```python
from build123d import *

# Parameters (mm, degrees)
F3_DEPTH = 82.392052


with BuildPart() as f1:
    # F0 (on Front) → F1 (revolve)
    with BuildSketch(Plane.XZ):
        with BuildLine():
            Line((-57.507594, 8), (-62.5, 8))
            Line((-62.5, 8), (-62.5, 0))
            Line((-62.5, 0), (-20.108948, 0))
            Line((-20.108948, 0), (19.891052, 0))
            Line((19.891052, 0), (62.5, 0))
            Line((62.5, 0), (62.5, 8))
            Line((62.5, 8), (57.492453, 8))
            Line((57.492453, 8), (57.492453, 5))
            Line((57.492453, 5), (52.492453, 5))
            Line((52.492453, 5), (52.492453, 8))
            Line((52.492453, 8), (19.891052, 8))
            Line((19.891052, 8), (19.891052, 96))
            ThreePointArc((19.891052, 96), (18.426586, 99.535534), (14.891052, 101))
            Line((14.891052, 101), (-15.108948, 101))
            ThreePointArc((-15.108948, 101), (-18.644481, 99.535534), (-20.108948, 96))
            Line((-20.108948, 96), (-20.108948, 8))
            Line((-20.108948, 8), (-52.507594, 8))
            Line((-52.507594, 8), (-52.507594, 5))
            Line((-52.507594, 5), (-57.507594, 5))
            Line((-57.507594, 5), (-57.507594, 8))
        make_face()
    revolve(axis=Axis((-6.764503, 0, 0), (1, 0, 0)))

    # F2 (on face) → F3 (cut, through all)
    with BuildSketch(Plane.YZ.offset(19.891052)):
        with BuildLine():
            Line((-9.635893, 76.123558), (-1.004641, 7.936668))
            ThreePointArc((-1.004641, 7.936668), (0, 8), (1.004641, 7.936668))
            Line((1.004641, 7.936668), (9.635893, 76.123558))
            Line((9.635893, 76.123558), (0, 76.123558))
            Line((0, 76.123558), (-9.635893, 76.123558))
        make_face()
    extrude(amount=-F3_DEPTH, mode=Mode.SUBTRACT)


solid = f1.part
```
CAD build for the part. Positions are in the model's coordinates, mm. A direction names the side the tool comes from. Coordinates: 2 decimals unless noted, no trailing zeros. Loops run counter-clockwise (first coordinate to the right, second up) from the corner with the lowest first, then second, coordinate; pieces in that order, holes last. Notation, with made-up numbers: (-40, -35) - (-33, -35) arc R27 cw to (-33, -10) - close; hole circle Ø2 at (-16.5, -27.5). An arc over 180 degrees is marked (long way). Use CSV: the item, a comma, the result in double quotes. Start each with the question number.
Q1. Cut at B-B, the plane x = 9.5. List the corners of the cut face in (y, z).
Q2. 3-axis set-ups, long thin cutter, end or side, ignore diameter. For faces 4 (the cylindrical face through (35.96, 7.81, -1.73)), 5 (the flat face through (-57.508, 5.2, 0.1)), 6 (the flat face through (0, 0, 76.124)), 7 (the cylindrical face through (-36.54, 7.81, -1.73)), 8 (the flat face through (62.5, 0, 0)): which of +Z, -Z, +X, -X, +Y, -Y reach the whole face in a straight line?
Q3. Drop flat-ended pins along their axis: P1, Ø4, axis at y = -76, z = -22, coming from the +X side; P2, Ø6, axis at y = -28, z = -80, coming from the -X side; P3, Ø1.5, axis at x = 36, z = 0.5, coming from the -Y side. Give the stop position or say it passes through.
Q4. Probe probe 1 along X at (y, z) = (3, 7); probe 2 along X at (y, z) = (-36.5, -22); probe 3 along Y at (x, z) = (14.5, 60). List the from-to ranges inside material, lowest first. Write a range as from..to.
Q5. Cut at C-C, the plane x = -32. List the corners of the cut face in (y, z).
Q6. Two-plate mould, pull along X, no slides. Class faces 1 (the flat face through (19.891, -1, -20)), 2 (the flat face through (0.17, -5.38, 42.51)), 3 (the flat face through (57.492, 5.2, -0.1)): +X half, -X half, draft (parallel to the pull), parting line (faces both ways), or undercut.
Here are the results:
1,outline,"circle Ø202 at (0, 0); hole (-9.64, 76.12) - (-1, 7.94) arc R8 cw to (1, 7.94) - (9.64, 76.12) - close"
2,face 4,"+X"
2,face 5,"none"
2,face 6,"+X, -X"
2,face 7,"-X"
2,face 8,"+Z, -Z, +X, +Y, -Y"
3,P1,"x = 19.89"
3,P2,"x = -20.11"
3,P3,"y = -8"
4,probe 1,"-62.5..-57.51, -52.51..52.49, 57.49..62.5"
4,probe 2,"-20.11..19.89"
4,probe 3,"-81.25..-7.59, 7.59..81.25"
5,outline,"circle Ø16 at (0, 0)"
6,face 1,"+X half"
6,face 2,"draft"
6,face 3,"undercut"
